Can you work these out from the drawing? Everything is in mm from the part's minimum corner. Coordinates: 2 decimals unless noted, no trailing zeros. Order: outer loops, then holes, each group sorted by start corner. A loop starts at its lowest first (then second) coordinate and runs counter-clockwise, first axis right, second up. Notation, with made-up numbers: M 10,41 L 41,41 A9 ccw 41,55 Z; hole C 42.25,73 d2. An arc over 180 degrees is marked long. Answer as a JSON object with one key per item and string values.
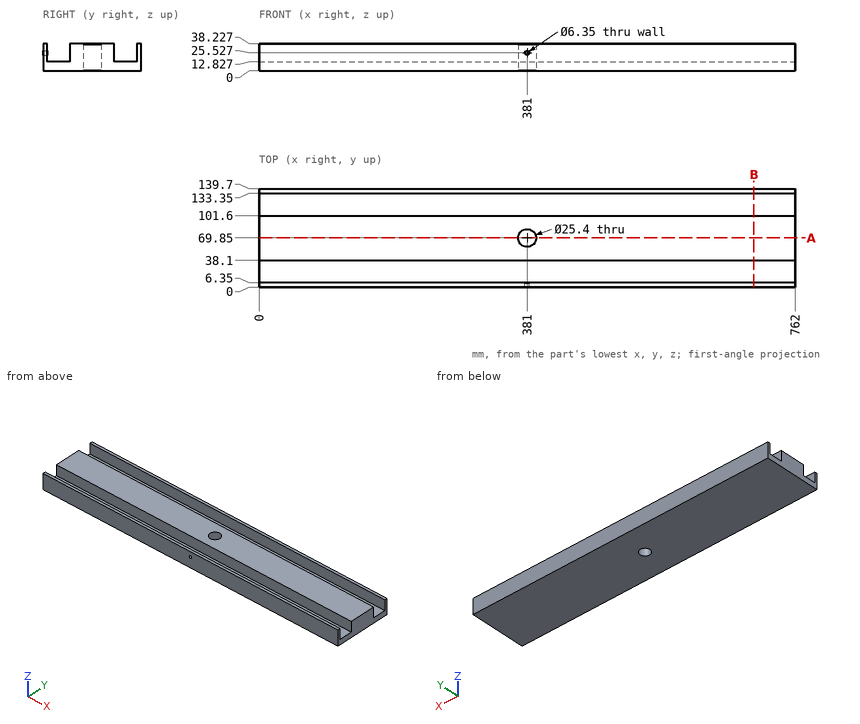
Item 1: Please list where these lines run through material, in increasing order: line 1 (Y direction, x = 667, z = 17); line 2 (Y direction, x = 381, z = 20).
Answers follow:
{"line 1": "y = 0 to 6.35, 38.1 to 101.6, 133.35 to 139.7", "line 2": "y = 0 to 6.35, 38.1 to 57.15, 82.55 to 101.6, 133.35 to 139.7"}
Item 2: I'm going to push a flat-ended pin straight in: pin 1 (3 mm diameter, centred on x = 355.5, z = 10, fed in from -Y). Where does the tip first touch, or does it pass through?
Answers follow:
{"pin 1": "stops at y = 0"}
Item 3: I want a section at A-A, the plane y = 69.85. Write out the boundary of the cut face in (x, z), plus the area to 3 significant figures.
Answers follow:
{"outline": "M 0,0 L 368.3,0 L 368.3,38.23 L 0,38.23 Z; M 393.7,0 L 762,0 L 762,38.23 L 393.7,38.23 Z", "area": "28,200 mm^2"}
Item 4: I want a section at B-B, the plane x = 703.5. Write out the boundary of the cut face in (y, z), plus the area to 3 significant figures.
Answers follow:
{"outline": "M 0,0 L 139.7,0 L 139.7,38.23 L 133.35,38.23 L 133.35,12.83 L 101.6,12.83 L 101.6,38.23 L 38.1,38.23 L 38.1,12.83 L 6.35,12.83 L 6.35,38.23 L 0,38.23 Z", "area": "3,730 mm^2"}
